Here's the drawing with two shaded views (mm, measured from the low corner). I have some questions. A direction names the side the tool comes from. Round coordinates to 2 decimals unless told otherwise and drop trailing zeros. Loops run counter-clockwise (first coordinate to the right, second up) from the corner with the lowest first, then second, coordinate; pieces in that order, holes last. Notation, with made-up numbers: (-8, 79) - (42, 79) arc R31 ccw to (42, 117) - close; hole circle Ø6 at (-24, -17.5). An arc over 180 degrees is marked (long way). Use one line per item in the form item = value.
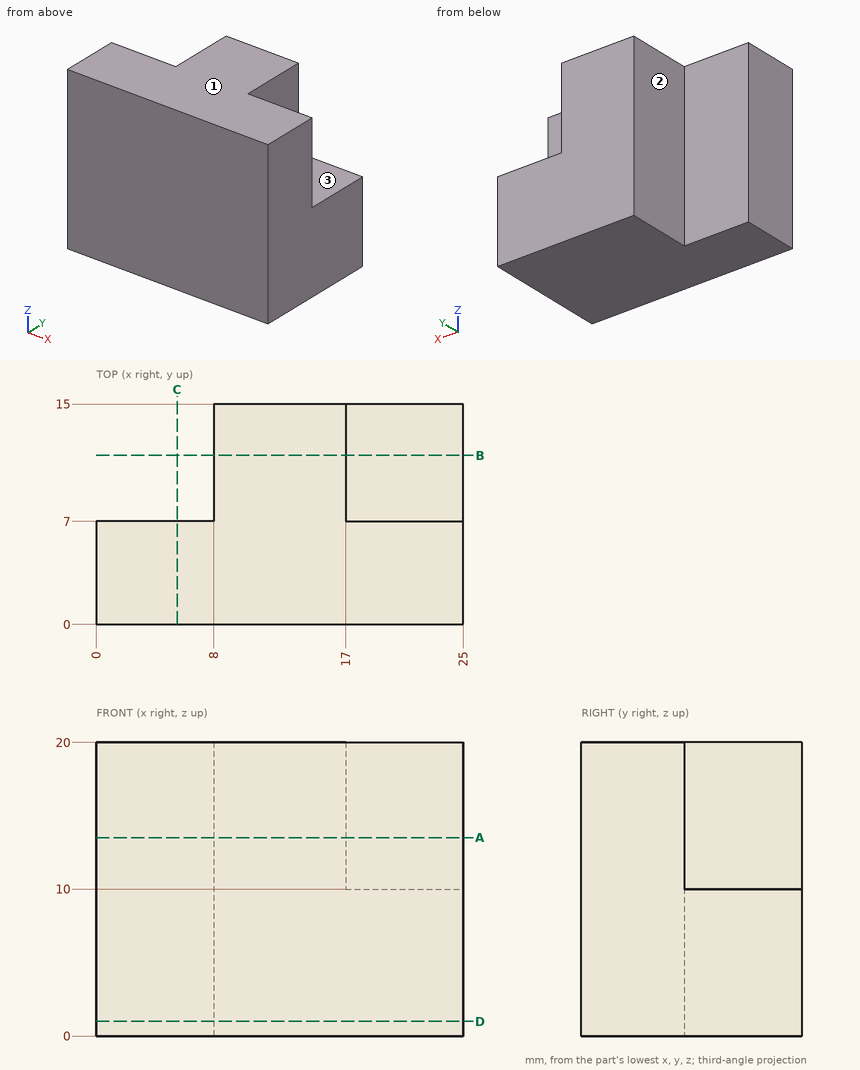
1. Please list where these lines run through material, in increasing order: line 1 along Y through (x, z) = (4.25, 3); line 2 along X through (y, z) = (11, 6); line 3 along X through (y, z) = (9, 13).
Solution:
line_1 = 0 to 7
line_2 = 8 to 25
line_3 = 8 to 17
2. If we section it at C-C, the plane x = 5.5: Write out the boundary of the cut face in (y, z), plus the area to 3 significant figures.
Solution:
outline = (0, 0) - (7, 0) - (7, 20) - (0, 20) - close
area = 140 mm^2
3. On a 3-axis mill with a long thin cutter (end or side, diameter ignored), from which of +Z, -Z, +X, -X, +Y, -Y can I reach the whole of each face in a straight line? I mean the marked faces 1, 2 and 3. Say none if no direction works.
Solution:
face_1 = +Z, +X, -X, +Y, -Y
face_2 = +Z, -Z, -X, +Y
face_3 = +Z, +X, +Y
4. If we section it at B-B, the plane y = 11.5: Write out the boundary of the cut face in (x, z).
Solution:
outline = (8, 0) - (25, 0) - (25, 10) - (17, 10) - (17, 20) - (8, 20) - close
5. If we section it at D-D, the plane z = 1: Write out the boundary of the cut face in (x, y).
Solution:
outline = (0, 0) - (25, 0) - (25, 15) - (8, 15) - (8, 7) - (0, 7) - close
6. If we section it at A-A, the plane z = 13.5: Write out the boundary of the cut face in (x, y).
Solution:
outline = (0, 0) - (25, 0) - (25, 7) - (17, 7) - (17, 15) - (8, 15) - (8, 7) - (0, 7) - close
7. For P1, Ø2, axis at y = 12.5, z = 13, coming from the +X side; P2, Ø1, axis at x = 21, y = 9.5, coming from the -Z side; P3, Ø4, axis at y = 10, z = 5, coming from the -X side; P4, Ø6.5, axis at x = 3, z = 11, coming from the +Y side, each with a flat end and sliding along its axis, tell me the tip position at first contact or that it passes through.
Solution:
P1 = 17
P2 = 0
P3 = 8
P4 = 7
